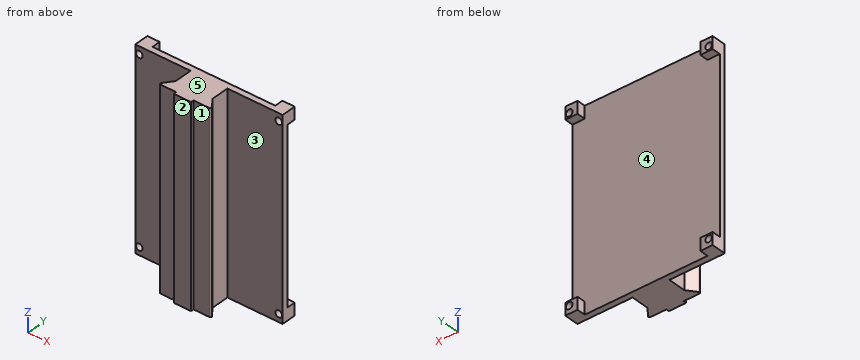
```python
from build123d import *

# Parameters (mm, degrees)
BOSS_EXTRUDE1_DEPTH   = 101.6
SKETCH4_W             = 6.35
SKETCH4_H             = 88.9
CUT_EXTRUDE1_DEPTH    = 4.444119865
SKETCH5_W             = 6.35
SKETCH5_H             = 88.9
CUT_EXTRUDE2_DEPTH    = 4.444119865
F_4_CLEARANCE_HOLE1_D = 3.4544
F_4_CLEARANCE_HOLE2_D = 3.4544
F_4_CLEARANCE_HOLE3_D = 3.4544
F_4_CLEARANCE_HOLE4_D = 3.4544


with BuildPart() as part:
    # Sketch1 → Boss-Extrude1 (new body)
    with BuildSketch(Plane.XY):
        with BuildLine():
            Line((-9.525, 2.8575), (-9.525, 4.453010906))
            Line((-9.525, 4.453010906), (-9.525, 12.073010906))
            Line((-9.525, 12.073010906), (-38.1, 12.073010906))
            Line((-38.1, 12.073010906), (-38.1, 19.568949913))
            Line((-38.1, 19.568949913), (-31.75, 19.568949913))
            Line((-31.75, 19.568949913), (-31.75, 15.124830048))
            Line((-31.75, 15.124830048), (31.75, 15.124830048))
            Line((31.75, 15.124830048), (31.75, 19.568949913))
            Line((31.75, 19.568949913), (38.1, 19.568949913))
            Line((38.1, 19.568949913), (38.1, 12.073010906))
            Line((38.1, 12.073010906), (9.525, 12.073010906))
            Line((9.525, 12.073010906), (9.525, 4.453010906))
            Line((9.525, 4.453010906), (9.525, 2.8575))
            Line((9.525, 2.8575), (13.126400516, -1.835936531))
            ThreePointArc((13.126400516, -1.835936531), (13.192135312, -2.503353309), (12.622621186, -2.8575))
            Line((12.622621186, -2.8575), (9.525, -2.8575))
            Line((9.525, -2.8575), (4.445, -2.8575))
            Line((4.445, -2.8575), (4.445, -4.3815))
            Line((4.445, -4.3815), (-4.445, -4.3815))
            Line((-4.445, -4.3815), (-4.445, -2.8575))
            Line((-4.445, -2.8575), (-9.525, -2.8575))
            Line((-9.525, -2.8575), (-12.622621186, -2.8575))
            ThreePointArc((-12.622621186, -2.8575), (-13.192135312, -2.503353309), (-13.126400516, -1.835936531))
            Line((-13.126400516, -1.835936531), (-9.525, 2.8575))
        make_face()
    extrude(amount=BOSS_EXTRUDE1_DEPTH)

    # Sketch4 → Cut-Extrude1 (cut)
    with BuildSketch(Plane(origin=(0, 19.568949913, 0), x_dir=(1, 0, 0), z_dir=(0, 1, 0))):
        with Locations((-34.925, -50.8)):
            Rectangle(SKETCH4_W, SKETCH4_H)
    extrude(amount=-CUT_EXTRUDE1_DEPTH, mode=Mode.SUBTRACT)

    # Sketch5 → Cut-Extrude2 (cut)
    with BuildSketch(Plane(origin=(0, 19.568949913, 0), x_dir=(1, 0, 0), z_dir=(0, 1, 0))):
        with Locations((34.925, -50.8)):
            Rectangle(SKETCH5_W, SKETCH5_H)
    extrude(amount=-CUT_EXTRUDE2_DEPTH, mode=Mode.SUBTRACT)

    # #4 Clearance Hole1 (through all)
    with Locations(Plane(origin=(-36.03625, 19.568949913, 3.96875), x_dir=(0, 0, 1), z_dir=(0, 1, 0))):
        with Locations((0, 0)):
            Hole(F_4_CLEARANCE_HOLE1_D / 2)

    # #4 Clearance Hole2 (through all)
    with Locations(Plane(origin=(36.03625, 19.568949913, 3.96875), x_dir=(0, 0, 1), z_dir=(0, 1, 0))):
        with Locations((0, 0)):
            Hole(F_4_CLEARANCE_HOLE2_D / 2)

    # #4 Clearance Hole3 (through all)
    with Locations(Plane(origin=(-36.03625, 19.568949913, 97.63125), x_dir=(0, 0, 1), z_dir=(0, 1, 0))):
        with Locations((0, 0)):
            Hole(F_4_CLEARANCE_HOLE3_D / 2)

    # #4 Clearance Hole4 (through all)
    with Locations(Plane(origin=(36.03625, 19.568949913, 97.63125), x_dir=(0, 0, 1), z_dir=(0, 1, 0))):
        with Locations((0, 0)):
            Hole(F_4_CLEARANCE_HOLE4_D / 2)


solid = part.part
```
Here's how the part is built. I have some questions about the finished solid (model axes, mm). Face numbers are marked on the shaded views. A direction names the side the tool comes from. Coordinates: 2 decimals unless noted, no trailing zeros. Order: outer loops, then holes, each group sorted by start corner. A loop starts at its lowest first (then second) coordinate and runs counter-clockwise, first axis right, second up.
1) Imagine slicing it at C-C on x = 21. List the corners of the cut face in (y, z) for me.
2) I need wall thicknesses on line 1 (Z direction, x = 35, y = 17); line 2 (X direction, y = 13.5, z = 5); line 3 (Y direction, x = -14, z = 28). Which ranges of each line are inside material? Lowest first, please.
3) Imagine slicing it at B-B on y = 17.5. List the corners of the cut face in (x, z) for me.
4) Imagine slicing it at A-A on z = 9. List the corners of the cut face in (x, y) for me (1 decimal), and give its area (3 significant figures).
5) Which directions (+Z, -Z, +X, -X, +Y, -Y) give clear straight access to the entire face, cutting with the end or side of a thin tool? Please do the marked faces 1 and 2.
6) Imagine slicing it at D-D on y = 9.25. List the corners of the cut face in (x, z) for me (3 decimals), and give its area (3 significant figures).
7) We'd pull the mould along Z, two halves only. Please class the marked faces 3, 4 and 5: +Z half, -Z half, draft (parallel to the pull), parting line (faces both ways), or undercut.
8) Will these pins go through, and if not, where does the flat tip stop? pin 1 (0.5 mm diameter, centred on y = -3.5, z = 44, fed in from -X) (3 decimals); pin 2 (23 mm diameter, centred on x = 21.5, z = 57.5, fed in from -Y); pin 3 (2 mm diameter, centred on x = -13.5, y = 0.5, fed in from -Z); pin 4 (8 mm diameter, centred on x = 3.5, z = 66, fed in from +Y).
Response values:
1. outline: (12.07, 0) - (15.12, 0) - (15.12, 101.6) - (12.07, 101.6) - close
2. line 1: z = 0 to 2.59, 5.35 to 6.35, 95.25 to 96.25, 99.01 to 101.6
2. line 2: x = -38.1 to -37.42, -34.65 to 34.65, 37.42 to 38.1
2. line 3: y = 12.07 to 15.12
3. outline: (-38.1, 0) - (-31.75, 0) - (-31.75, 6.35) - (-38.1, 6.35) - close; (-38.1, 95.25) - (-31.75, 95.25) - (-31.75, 101.6) - (-38.1, 101.6) - close; (31.75, 0) - (38.1, 0) - (38.1, 6.35) - (31.75, 6.35) - close; (31.75, 95.25) - (38.1, 95.25) - (38.1, 101.6) - (31.75, 101.6) - close; hole circle Ø3.45 at (-36.04, 3.97); hole circle Ø3.45 at (-36.04, 97.63); hole circle Ø3.45 at (36.04, 3.97); hole circle Ø3.45 at (36.04, 97.63)
4. outline: (-38.1, 12.1) - (-9.5, 12.1) - (-9.5, 2.9) - (-13.1, -1.8) arc R0.6 ccw to (-12.6, -2.9) - (-4.4, -2.9) - (-4.4, -4.4) - (4.4, -4.4) - (4.4, -2.9) - (12.6, -2.9) arc R0.6 ccw to (13.1, -1.8) - (9.5, 2.9) - (9.5, 12.1) - (38.1, 12.1) - (38.1, 15.1) - (-38.1, 15.1) - close
4. area: 555 mm2
5. face 1: +Z, -Z, +X, -Y
5. face 2: +Z, -Z, +X, -X, -Y
6. outline: (-9.525, 0) - (9.525, 0) - (9.525, 101.6) - (-9.525, 101.6) - close
6. area: 1,940 mm2
7. face 3: draft
7. face 4: undercut
7. face 5: +Z half
8. pin 1: stops at x = -4.445
8. pin 2: stops at y = -2.86
8. pin 3: passes through
8. pin 4: stops at y = 15.12
